from build123d import *

# Parameters (mm, degrees)
SKETCH1_R           = 2
BOSS_EXTRUDE1_DEPTH = 3
BOSS_EXTRUDE2_DEPTH = 0.15
CIRPATTERN1_COUNT   = 2


with BuildPart() as part:
    # Sketch1 → Boss-Extrude1 (new body)
    with BuildSketch(Plane(origin=(0, 0, 0), x_dir=(1, 0, 0), z_dir=(0, 1, 0))):
        with Locations(Location((0, 0, 0), (0, 0, 270))):
            Circle(SKETCH1_R)
    extrude(amount=BOSS_EXTRUDE1_DEPTH)

    # Sketch3 → Boss-Extrude2 (add, symmetric)
    with BuildSketch(Plane(origin=(0.574533332, 1.232090707, 0), x_dir=(0.9063077870366496, -0.4226182617407003, 0), z_dir=(-0.42261826174070033, -0.9063077870366497, 0))):
        with BuildLine():
            Line((-1.825963844, 0), (-2.618118511, 0.610320395))
            Line((-2.618118511, 0.610320395), (-2.618118511, 13.644717252))
            ThreePointArc((-2.618118511, 13.644717252), (-2.325225292, 14.351824033), (-1.618118511, 14.644717252))
            Line((-1.618118511, 14.644717252), (-1.229872287, 14.644717252))
            ThreePointArc((-1.229872287, 14.644717252), (0.676144985, 13.961417094), (1.713907655, 12.222782692))
            add(Edge.make_bspline(
                [(1.572828445, 0), (2.462700646, 4.059259168), (2.506395313, 8.187064394), (1.713907655, 12.222782692)],
                knots=[0, 0, 0, 0, 0.833038136, 0.833038136, 0.833038136, 0.833038136], degree=3))
            Line((1.572828445, 0), (-1.825963844, 0))
        make_face()
    boss_extrude2 = extrude(amount=BOSS_EXTRUDE2_DEPTH, both=True)

    # CirPattern1: Boss-Extrude2 ×2 about axis
    cirpattern1_axis = Axis((0, 3.15, 0), (0, -1, 0))
    for i in range(1, CIRPATTERN1_COUNT):
        add(boss_extrude2.rotate(cirpattern1_axis, i * 360 / CIRPATTERN1_COUNT))


solid = part.part
The model under review builds one solid part; all positions refer to its coordinate system, in mm. A direction names the side the tool comes from. Coordinates: 2 decimals unless noted, no trailing zeros.
(1) Wall thickness on L1, parallel to Z at x = -0.65, y = 0.7; L2, parallel to X at y = 1.55, z = 9; L3, parallel to Z at x = -0.1, y = 0.55: over which ranges is each line inside the solid? List them lowest first.
Determined:
L1: z = -1.89 to 1.89
L2: x = -0.46 to 0.25
L3: z = -2 to 2
(2) Tool access review of faces 1 (the cylindrical face through (-0.766, 1.479, 1.847)), 2 (the flat face through (0, 0, 0)): name each direction out of +Z, -Z, +X, -X, +Y, -Y from which nothing blocks a thin tool from reaching the whole face with its end or side.
Determined:
face 1: none
face 2: +Z, -Z, +X, -X, -Y
(3) Insertion check: P1, Ø1, axis at x = 0, z = -5, coming from the +Y side; P2, Ø2, axis at x = -2, z = -11, coming from the +Y side; P3, Ø2, axis at x = 0.5, z = -11.5, coming from the +Y side. Each pin has a flat end and moves straight along its axis. Give the tip position at first contact, or say it passes through.
Determined:
P1: stops at y = 1.9
P2: stops at y = 1.2
P3: stops at y = 2.36
